Could you check a few things on this model? Use its own coordinates, in mm. Give positions to 0.01 mm unless a question says otherwise; leave off trailing zeros. Write each loop counter-clockwise with the first axis right and the second up, starting at its lowest first coordinate (ties: lowest second). Pieces come first, ordered by that corner, then holes. Notation, with made-up numbers: M 38.5,72.25 L 57.5,72.25 A29 cw 57.5,103.25 Z; hole C 79,38.25 d9. An arc over 180 degrees is marked long. Answer as CSV lines item,"result". Start each with the question number.
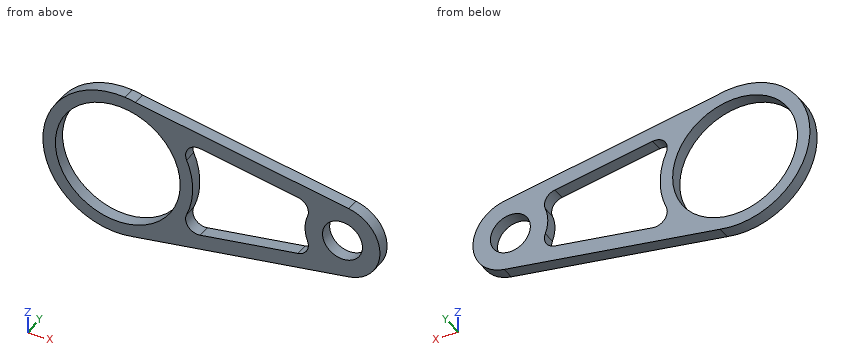
from build123d import *

# Parameters (mm, degrees)
F0_R     = 25
F0_R_2   = 8
F1_DEPTH = 5


with BuildPart() as f1:
    # F0 (on Front) → F1 (new body)
    with BuildSketch(Plane.XZ):
        with BuildLine():
            Line((2.888273, 29.860641), (7.037978, 29.162765))
            ThreePointArc((7.037978, 29.162765), (4.975377, 29.584551), (2.888273, 29.860641))
        make_face()
        with BuildLine():
            Line((92.487688, 14.792275), (7.037978, 29.162765))
            Line((7.037978, 29.162765), (2.888273, 29.860641))
            ThreePointArc((2.888273, 29.860641), (-29.958665, -1.5743), (6.002022, -29.393464))
            Line((6.002022, -29.393464), (92.49708, -14.790693))
            ThreePointArc((92.49708, -14.790693), (104.999999, 0.004762), (92.487688, 14.792275))
        make_face()
        with BuildLine():
            ThreePointArc((27.576515, 11.812529), (28.24219, 16.871895), (33.00183, 18.712042))
            Line((33.00183, 18.712042), (72.168065, 12.125267))
            ThreePointArc((72.168065, 12.125267), (75.682636, 9.670676), (76.004127, 5.395882))
            ThreePointArc((76.004127, 5.395882), (75.000001, -0.004762), (76.007556, -5.404768))
            ThreePointArc((76.007556, -5.404768), (75.688779, -9.679765), (72.175768, -12.136588))
            Line((72.175768, -12.136588), (32.987291, -18.752693))
            ThreePointArc((32.987291, -18.752693), (28.223524, -16.911805), (27.561369, -11.847824))
            ThreePointArc((27.561369, -11.847824), (29.999994, -0.019204), (27.576515, 11.812529))
        make_face(mode=Mode.SUBTRACT)
        Circle(F0_R, mode=Mode.SUBTRACT)
        with Locations((90, 0)):
            Circle(F0_R_2, mode=Mode.SUBTRACT)
    extrude(amount=F1_DEPTH)


solid = f1.part
1. Imagine slicing it at D-D, the plane z = -22.5. Please give me the cut outline in (x, y).
2. Imagine slicing it at B-B, the plane x = 0. Please give me the cut outline in (y, z).
3. Will these pins go through, and if not, where does the flat tip stop? P1, Ø1.5, axis at x = 1.5, y = -1, coming from the -Z side; P2, Ø1, axis at x = 74.5, y = -2.5, coming from the -Z side; P3, Ø1, axis at y = -2, z = 6, coming from the -X side.
4. Please list where these lines run through material, in increasing order: line 1 (Z direction, x = 0, y = -1.9); line 2 (X direction, y = -1.45, z = -10); line 3 (X direction, y = -2.6, z = -2.5).
5. Imagine slicing it at C-C, the plane y = -2.05. Please give me the cut outline in (x, z).
6. Imagine slicing it at A-A, the plane z = 0. Please give me the cut outline in (x, y), plus the area to 3 significant figures.
Solutions:
1,outline,"M -19.84,-5 L -10.9,-5 L -10.9,0 L -19.84,0 Z; M 10.9,-5 L 46.83,-5 L 46.83,0 L 10.9,0 Z"
2,outline,"M -5,-30 L 0,-30 L 0,-25 L -5,-25 Z; M -5,25 L 0,25 L 0,30 L -5,30 Z"
3,P1,"z = -29.99"
3,P2,"z = -17.91"
3,P3,"x = -29.49"
4,line 1,"-30 to -25, 25 to 30"
4,line 2,"-28.28 to -22.91, 22.91 to 28.28, 75.49 to 101.18"
4,line 3,"-29.9 to -24.87, 24.87 to 29.9, 75.21 to 82.4, 97.6 to 104.79"
5,outline,"M 2.89,29.86 A30 ccw long 6,-29.39 L 92.5,-14.79 A15 ccw 92.49,14.79 L 7.04,29.16 A30 ccw Z; hole C 0,0 d50; hole M 27.56,-11.85 A5 ccw 32.99,-18.75 L 72.18,-12.14 A5 ccw 76.01,-5.4 A15 cw 76,5.4 A5 ccw 72.17,12.13 L 33,18.71 A5 ccw 27.58,11.81 A30 cw Z; hole C 90,0 d16"
6,outline,"M -30,-5 L -25,-5 L -25,0 L -30,0 Z; M 25,-5 L 30,-5 L 30,0 L 25,0 Z; M 75,-5 L 82,-5 L 82,0 L 75,0 Z; M 98,-5 L 105,-5 L 105,0 L 98,0 Z"
6,area,"120 mm²"
